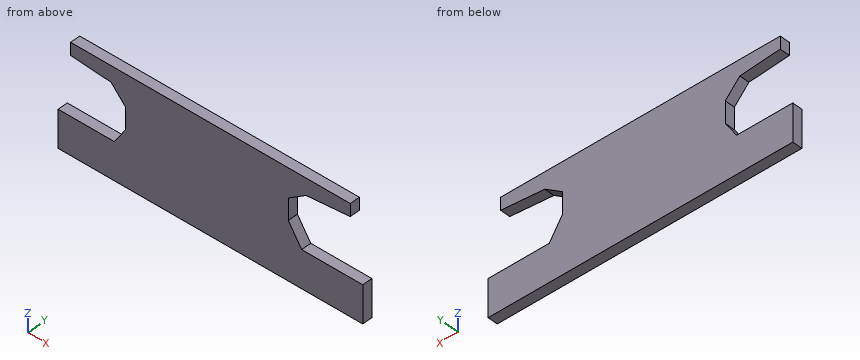
```python
from build123d import *

# Parameters (mm, degrees)
SKETCH1_W         = 48.84
SKETCH1_H         = 17.34
MAIN_SQUARE_DEPTH = 1.6
SERVO_HOLES_DEPTH = 1.6


with BuildPart() as part:
    # Sketch1 → main square (new body)
    with BuildSketch(Plane(origin=(0, 0, 0), x_dir=(1, 0, 0), z_dir=(0, 1, 0))):
        with Locations((24.42, 8.67)):
            Rectangle(SKETCH1_W, SKETCH1_H)
    extrude(amount=MAIN_SQUARE_DEPTH)

    # Sketch2 → servo holes (cut)
    with BuildSketch(Plane(origin=(0, 1.6, 0), x_dir=(1, 0, 0), z_dir=(0, 1, 0))):
        Polygon((46.84, 2), (46.84, 0), (48.84, 0), (48.84, 11.34), (39.04, 11.34), (36.91, 8.061097745), (36.91, 4.611097745), (39.750024568, 2.67), align=None)
        Polygon((9, 11.34), (0, 11.34), (0, 0), (2, 0), (2, 2), (8.486484798, 2.55), (10.82, 5.07751), (10.82, 8.52751), align=None)
    extrude(amount=-SERVO_HOLES_DEPTH, mode=Mode.SUBTRACT)


solid = part.part
```
Geometry: final body of the model. Coordinates: model frame, mm. Round coordinates to 2 decimals unless told otherwise and drop trailing zeros. Order: outer loops, then holes, each group sorted by start corner. A loop starts at its lowest first (then second) coordinate and runs counter-clockwise, first axis right, second up. Notation, with made-up numbers: M -31,-34 L 4,-34 A11 ccw 4,-24 Z; hole C 26.25,-27.75 d7. An arc over 180 degrees is marked long. Use one line per item in the form item = value. Start each with the question number.
Q1. Cut plane D-D (x = 44.5). Return loops of the section in (y, z), and give its area (3 significant figures).
Q2. Cut plane A-A (x = 38). Return loops of the section in (y, z).
Q3. Material intervals for line 1 (X direction, y = 0.15, z = -7.25); line 2 (X direction, y = 1.2, z = -1.25), sorted ascending. Write a range as [from, to].
Q4. Pin query (flat end, axial travel): pin 1 Ø0.8 at (y, z) = (0.5, -1) entering from -X; pin 2 Ø5 at (x, z) = (6, -6) entering from +Y; pin 3 Ø0.8 at (y, z) = (1, -6.5) entering from -X; pin 4 Ø0.8 at (y, z) = (1, -1) entering from +X. Return the tip coordinate at first contact, or that it passes through.
Q5. Cut plane B-B (y = 0.6). Return loops of the section in (x, z), and give its area (3 significant figures).
Q6. Cut plane C-C (z = -1.5). Return loops of the section in (x, y), and give its area (3 significant figures).
Geometry results:
q1.outline = M 0,-17.34 L 1.6,-17.34 L 1.6,-11.34 L 0,-11.34 Z; M 0,-2.22 L 1.6,-2.22 L 1.6,0 L 0,0 Z
q1.area = 13.2 mm^2
q2.outline = M 0,-17.34 L 1.6,-17.34 L 1.6,-9.74 L 0,-9.74 Z; M 0,-3.87 L 1.6,-3.87 L 1.6,0 L 0,0 Z
q3.line_1 = [10.82, 36.91]
q3.line_2 = [2, 46.84]
q4.pin_1 = 2
q4.pin_2 = through
q4.pin_3 = 10.82
q4.pin_4 = 46.84
q5.outline = M 0,-17.34 L 48.84,-17.34 L 48.84,-11.34 L 39.04,-11.34 L 36.91,-8.06 L 36.91,-4.61 L 39.75,-2.67 L 46.84,-2 L 46.84,0 L 2,0 L 2,-2 L 8.49,-2.55 L 10.82,-5.08 L 10.82,-8.53 L 9,-11.34 L 0,-11.34 Z
q5.area = 646 mm^2
q6.outline = M 2,0 L 46.84,0 L 46.84,1.6 L 2,1.6 Z
q6.area = 71.7 mm^2
